Input: dimensioned drawing with shaded views. Units: mm. Origin: part minimum x, y, z. A direction names the side the tool comes from. Coordinates: 2 decimals unless noted, no trailing zeros. Order: outer loops, then holes, each group sorted by start corner. A loop starts at its lowest first (then second) coordinate and runs counter-clockwise, first axis right, second up. Notation, with made-up numbers: (-8, 60) -> (36, 60) arc R28 cw to (36, 84) -> close; hole circle Ø3 at (-22.75, -15). An arc over 180 degrees is marked (long way). Answer as CSV lines item,"result".
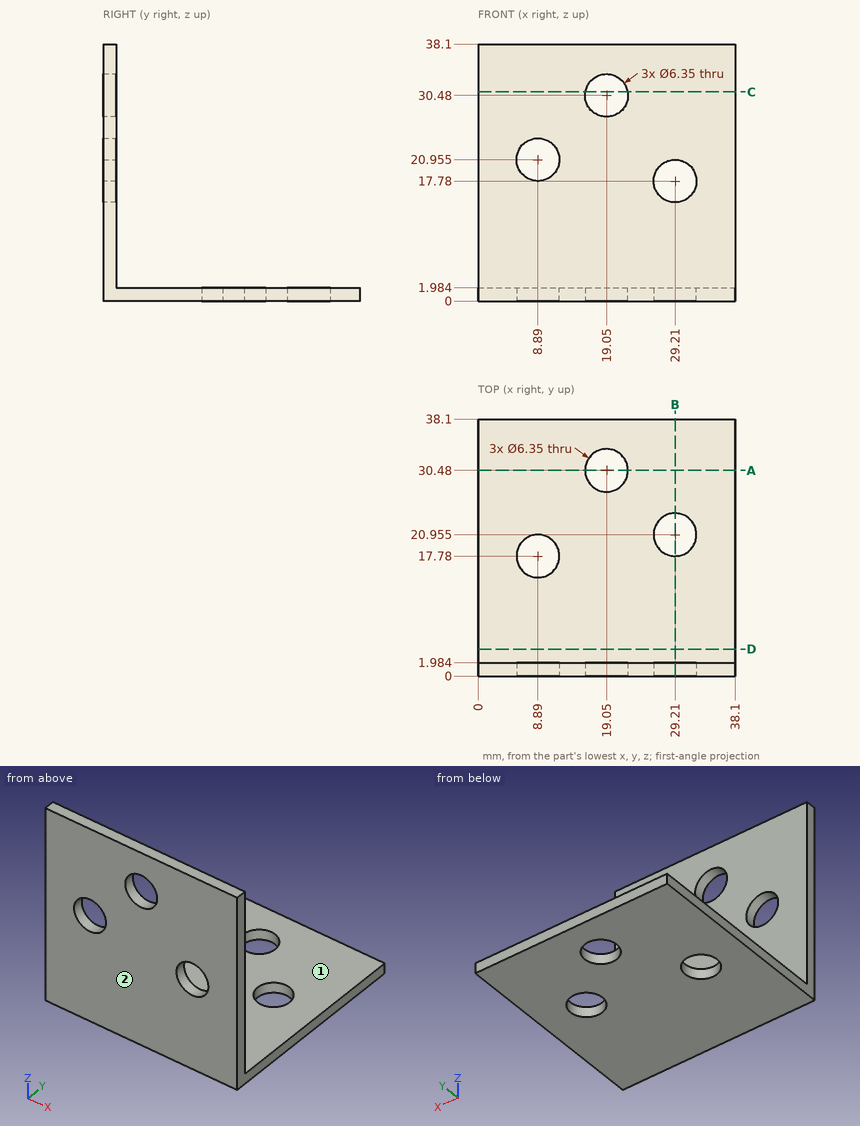
1. Contact query for flat-ended pins moving along their axis: pin 1 (5 mm diameter, centred on x = 8.89, y = 17.78, fed in from +Z); pin 2 (10 mm diameter, centred on x = 19.05, z = 30.48, fed in from +Y); pin 3 (1.5 mm diameter, centred on x = 21.5, y = 21, fed in from +Z). Output: stop coordinate, or through.
Findings:
pin 1,"passes through"
pin 2,"stops at y = 1.98"
pin 3,"stops at z = 1.98"
2. Cut plane A-A (y = 30.48). Return the cut outline in (x, z) (1 decimal).
Findings:
outline,"(0, 0) -> (15.9, 0) -> (15.9, 2) -> (0, 2) -> close; (22.2, 0) -> (38.1, 0) -> (38.1, 2) -> (22.2, 2) -> close"
3. Cut plane D-D (y = 4). Return the cut outline in (x, z) (1 decimal).
Findings:
outline,"(0, 0) -> (38.1, 0) -> (38.1, 2) -> (0, 2) -> close"
4. Ray query, line 1 along Y through (x, z) = (8.89, 0.9) (1 decimal); line 2 along Y through (x, z) = (29.21, 1.3); line 3 along Z through (x, y) = (34, 14) (1 decimal). Return the intervals inside material, ascending.
Findings:
line 1,"y = 0 to 14.6, 21 to 38.1"
line 2,"y = 0 to 17.78, 24.13 to 38.1"
line 3,"z = 0 to 2"
5. Reachability of the marked faces 1 and 2 from +Z, -Z, +X, -X, +Y, -Y: full face, straight path, thin tool, end or side. Return the list, or none.
Findings:
face 1,"+Z, +X, -X, +Y"
face 2,"+Z, -Z, +X, -X, -Y"
6. Cut plane B-B (x = 29.21). Return the cut outline in (y, z) (1 decimal), plus the area to 3 significant figures.
Findings:
outline,"(0, 0) -> (17.8, 0) -> (17.8, 2) -> (2, 2) -> (2, 14.6) -> (0, 14.6) -> close; (0, 21) -> (2, 21) -> (2, 38.1) -> (0, 38.1) -> close; (24.1, 0) -> (38.1, 0) -> (38.1, 2) -> (24.1, 2) -> close"
area,"122 mm2"
